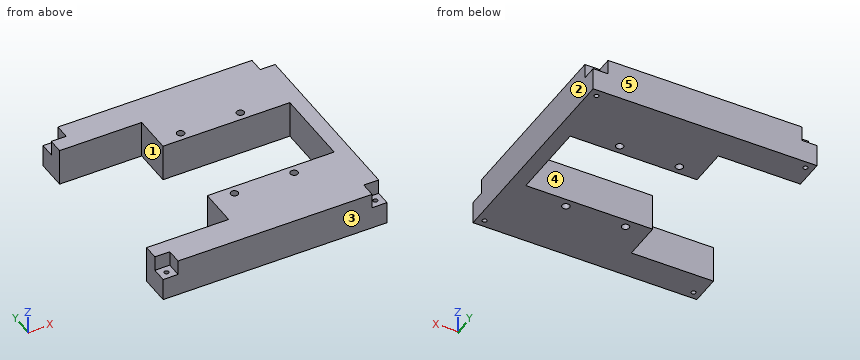
Autodesk Inventor part; units mm, degrees
ref_plane "YZ Plane" through (0, 0, 0) normal (1, 0, 0) x (0, 1, 0)
ref_plane "XZ Plane" through (0, 0, 0) normal (0, 1, 0) x (-1, 0, 0)
ref_plane "XY Plane" through (0, 0, 0) normal (0, 0, 1) x (1, 0, 0)
sketch "스케치1" plane through (0, 0, 0) normal (0, 0, 1) x (1, 0, 0)
  line L0 (0, 0) -> (300, 0)
  line L1 (300, 0) -> (300, 290)
  line L2 (300, 290) -> (0, 290)
  line L3 (0, 290) -> (0, 0)
  line L4 (300, 270) -> (245, 270)
  line L5 (245, 270) -> (245, 165)
  line L6 (245, 165) -> (300, 165)
  line L7 (300, 165) -> (300, 270)
  line L8 (150, 290) -> (150, 145)
  line L9 (0, 270) -> (55, 270)
  line L10 (55, 270) -> (55, 165)
  line L11 (55, 165) -> (0, 165)
  line L12 (300, 145) -> (150, 145)
  line L13 (300, 20) -> (245, 20)
  line L14 (245, 20) -> (245, 125)
  line L15 (245, 125) -> (300, 125)
  line L16 (55, 125) -> (0, 125)
  line L17 (55, 20) -> (55, 125)
  line L18 (0, 20) -> (55, 20)
  line L19 (0, 145) -> (150, 145)
  circle A0 centre (5, 150) radius 1.5
  circle A1 centre (145, 150) radius 1.5
  circle A2 centre (5, 285) radius 1.5
  circle A3 centre (145, 285) radius 1.5
  point P0 (300, 165)
  point P1 (0, 165)
  dimension "d0" = 290
  dimension "d1" = 300
  dimension "d12" = 105
  dimension "d13" = 55
  dimension "d14" = 20
  dimension "d18" = 5
  dimension "d19" = 3
  dimension "d20" = 5
  dimension "d21" = 5
  dimension "d22" = 5
extrude "돌출1" add sketch "스케치1" along normal blind 25 contours L3 L11 L10 L9 L2 L8 L19
sketch "스케치3" plane through (0, 0, 25) normal (0, 0, 1) x (1, 0, 0)
  line L0 (55, 165) -> (0, 165)
  line L1 (0, 165) -> (0, 145)
  line L2 (0, 145) -> (150, 145)
  line L3 (150, 145) -> (150, 290)
  line L4 (150, 290) -> (0, 290)
  line L5 (0, 290) -> (0, 270)
  line L6 (0, 270) -> (55, 270)
  line L7 (55, 270) -> (55, 165)
  circle A0 centre (145, 285) radius 1.5
  circle A1 centre (5, 285) radius 1.5
  circle A2 centre (145, 150) radius 1.5
  circle A3 centre (5, 150) radius 1.5
  line L8 (140, 145) -> (140, 290)
  line L9 (140, 155) -> (150, 155)
  line L10 (140, 280) -> (150, 280)
  line L11 (0, 155) -> (10, 155)
  line L12 (10, 155) -> (10, 145)
  line L13 (0, 280) -> (10, 280)
  line L14 (10, 280) -> (10, 290)
  point P0 (0, 0)
  dimension "d23" = 10
  dimension "d24" = 10
  dimension "d25" = 10
extrude "돌출3" cut sketch "스케치3" against normal blind 10 contours L11 L12 L2 L1 | L5 L4 L14 L13 | L8 L9 L3 L2 | L4 L3 L10 L8
sketch "스케치4" plane through (55, 165, 0) normal (-1, 0, 0) x (0, 0, 1)
  line L0 (22, 11) -> (22, 94)
  line L1 (22, 94) -> (0, 94)
  line L2 (0, 105) -> (0, 0)
  line L3 (0, 0) -> (25, 0)
  line L4 (25, 105) -> (25, 0)
  line L5 (0, 105) -> (25, 105)
  line L6 (22, 11) -> (0, 11)
  circle A0 centre (14.25, 17) radius 2.5
  circle A1 centre (14.25, 88) radius 2.5
  line L7 (0, 25.75) -> (0, 79.25)
  line L8 (0, 25.75) -> (25, 25.75)
  line L9 (0, 79.25) -> (25, 79.25)
  line L10 (6.5, 11) -> (6.5, 94)
  point P0 (0, -165)
  point P1 (22, 52.5)
  point P2 (25, 52.5)
  point P3 (0, 52.5)
  point P4 (6.5, 79.25)
  point P5 (22, 79.25)
  point P6 (6.5, 25.75)
  point P7 (22, 25.75)
  dimension "d28" = 83
  dimension "d30" = 5
  dimension "d31" = 5
  dimension "d33" = 6
  dimension "d34" = 6
  dimension "d35" = 53.5
  dimension "d36" = 15.5
  dimension "d37" = 7.75
  dimension "d39" = 3
extrude "돌출5" cut sketch "스케치4" against normal blind 85 contours L8 L10 L9 L0 | L0 L9 L4 L8 | L8 L2 L9 L10
sketch "스케치5" plane through (0, 0, 25) normal (0, 0, 1) x (1, 0, 0)
  line L0 (55, 244.25) -> (140, 244.25)
  line L1 (140, 244.25) -> (140, 190.75)
  line L2 (140, 190.75) -> (55, 190.75)
  line L3 (55, 190.75) -> (55, 165)
  line L4 (55, 165) -> (0, 165)
  line L5 (0, 165) -> (0, 155)
  line L6 (0, 155) -> (10, 155)
  line L7 (10, 155) -> (10, 145)
  line L8 (10, 145) -> (140, 145)
  line L9 (140, 145) -> (140, 155)
  line L10 (140, 155) -> (150, 155)
  line L11 (150, 155) -> (150, 280)
  line L12 (150, 280) -> (140, 280)
  line L13 (140, 280) -> (140, 290)
  line L14 (140, 290) -> (10, 290)
  line L15 (10, 290) -> (10, 280)
  line L16 (10, 280) -> (0, 280)
  line L17 (0, 280) -> (0, 270)
  line L18 (0, 270) -> (55, 270)
  line L19 (55, 270) -> (55, 244.25)
  circle A0 centre (70, 185) radius 2.5
  circle A1 centre (70, 250) radius 2.5
  circle A2 centre (110, 185) radius 2.5
  circle A3 centre (110, 250) radius 2.5
  point P0 (0, 0)
  point P1 (140, 217.5)
  dimension "d47" = 15
  dimension "d48" = 65
  dimension "d49" = 32.5
  dimension "d50" = 5
  dimension "d51" = 65
  dimension "d52" = 5
  dimension "d53" = 40
extrude "돌출7" cut sketch "스케치5" against normal through all contours A0 | A1 | A2 | A3
equation "\"d20\" = d18"
equation "\"d21\" = d20"
equation "\"d22\" = d21"
equation "\"d37\" = 0.5 * d36"
properties part number "RobotBase_3D 인쇄"
Read the model definition and answer for the solid it produces. Units are mm, in the model's axes. Face numbers are marked on the shaded views. A direction names the side the tool comes from. Give positions to 0.01 mm unless a question says otherwise; leave off trailing zeros. Write each loop counter-clockwise with the first axis right and the second up, starting at its lowest first coordinate (ties: lowest second). Pieces come first, ordered by that corner, then holes. Notation, with made-up numbers: M -15,35.5 L 41,35.5 A21 ccw 41,72.5 Z; hole C 36.25,-7 d11. An arc over 180 degrees is marked long. One line per item, written item: value. Start each with the question number.
(1) Determine the mould class of the marked faces 1, 2 and 3 for opening direction Y: pulls with the +Y half, pulls with the -Y half, needs draft (parallel to the pull), parting line crosses it, or undercut.
(2) Find the intervals of material crossed by line 1 (X direction, y = 285, z = 6); line 2 (Y direction, x = 35, z = 5); line 3 (Y direction, x = 86, z = 8), in increasing order.
(3) A tool of negligible diameter and unlimited length cuts with its end or side. For the marked faces 4 and 5, from which of +Z, -Z, +X, -X, +Y, -Y can it reach the whole face along a straight path? Write none if from no direction.
(4) Flat-ended cylindrical pins translate along their axes: pin 1 Ø1.8 at (x, y) = (5, 150) entering from +Z; pin 2 Ø7.5 at (y, z) = (178, 9.5) entering from -X; pin 3 Ø5 at (x, y) = (5, 286) entering from +Z; pin 4 Ø7.5 at (y, z) = (212.5, 6.5) entering from -X. Find the tip coordinate at first contact, or state that the pin passes through.
(5) Find section A-A (x = 59). Determine the outline of the cut face in (y, z), plus the area to 3 significant figures.
(6) Find section C-C (x = 110). Determine the outline of the cut face in (y, z), plus the area to 3 significant figures.
(7) Find section B-B (z = 6). Give the number of separate pieces and of enclosed holes in the cut face, plus the area to 3 significant figures.
(8) Find section D-D (y = 215). Determine the outline of the cut face in (x, z).
Results below:
1. face 1: undercut
1. face 2: needs draft
1. face 3: pulls with the -Y half
2. line 1: x = 0 to 3.5, 6.5 to 143.5, 146.5 to 150
2. line 2: y = 145 to 165, 270 to 290
2. line 3: y = 145 to 190.75, 244.25 to 290
3. face 4: +Z, -Z, -X
3. face 5: +Z, -Z, +X, -X, +Y
4. pin 1: passes through
4. pin 2: stops at x = 55
4. pin 3: stops at z = 15
4. pin 4: stops at x = 140
5. outline: M 145,0 L 190.75,0 L 190.75,25 L 145,25 Z; M 244.25,0 L 290,0 L 290,25 L 244.25,25 Z
5. area: 2,290 mm^2
6. outline: M 145,0 L 182.5,0 L 182.5,25 L 145,25 Z; M 187.5,0 L 190.75,0 L 190.75,25 L 187.5,25 Z; M 244.25,0 L 247.5,0 L 247.5,25 L 244.25,25 Z; M 252.5,0 L 290,0 L 290,25 L 252.5,25 Z
6. area: 2,040 mm^2
7. separate pieces: 1
7. enclosed holes: 8
7. area: 11,300 mm^2
8. outline: M 140,0 L 150,0 L 150,25 L 140,25 Z
